Design review of the part built by this model. Coordinates are the model's own, in mm. A direction names the side the tool comes from. Coordinates: 2 decimals unless noted, no trailing zeros. Loops run counter-clockwise (first coordinate to the right, second up) from the corner with the lowest first, then second, coordinate; pieces in that order, holes last. Notation, with made-up numbers: (30, 49.25) - (88, 49.25) arc R19 ccw to (88, 57.25) - close; hole circle Ø10 at (-19.75, 79.25). An arc over 180 degrees is marked (long way). One line per question, with ' | ' between items.
from build123d import *

# Parameters (mm, degrees)
SKETCH_1_W          = 15
SKETCH_1_H          = 15
SKETCH_1_W_2        = 12
SKETCH_1_H_2        = 12
EXTRUDE_1_DEPTH     = 780
CUT_EXTRUDE_1_REACH = 782.288
SKETCH_2_R          = 2.15
CUT_EXTRUDE_2_REACH = 782.288
SKETCH_4_R          = 2.15


with BuildPart() as part:
    # ｽｹｯﾁ1 → 押し出し-薄板1 (new body)
    with BuildSketch(Plane(origin=(0, 0, 0), x_dir=(1, 0, 0), z_dir=(0, 1, 0))):
        with Locations((7.5, 7.5)):
            Rectangle(SKETCH_1_W, SKETCH_1_H)
        with Locations((7.5, 7.5)):
            Rectangle(SKETCH_1_W_2, SKETCH_1_H_2, mode=Mode.SUBTRACT)
    extrude(amount=EXTRUDE_1_DEPTH)

    # ｶｯﾄ - 押し出し1: up to this face of the body (flat: up to its plane)
    cut_extrude_1_end = Plane(part.part.faces().sort_by_distance((0, 390, -7.5))[0])
    # ｽｹｯﾁ2 → ｶｯﾄ - 押し出し1 (cut, up to the picked face)
    with BuildSketch(Plane(origin=(15, 0, 0), x_dir=(0, 0, -1), z_dir=(1, 0, 0)), mode=Mode.PRIVATE) as cut_extrude_1_sk1:
        with Locations((7.5, 730)):
            Circle(SKETCH_2_R)
    cut_extrude_1_tool1 = split(extrude(cut_extrude_1_sk1.sketch, amount=-CUT_EXTRUDE_1_REACH, mode=Mode.PRIVATE), bisect_by=cut_extrude_1_end, keep=Keep.BOTH, mode=Mode.PRIVATE)
    # ｽｹｯﾁ2 → ｶｯﾄ - 押し出し1 (cut, up to the picked face)
    with BuildSketch(Plane(origin=(15, 0, 0), x_dir=(0, 0, -1), z_dir=(1, 0, 0)), mode=Mode.PRIVATE) as cut_extrude_1_sk2:
        with Locations((7.5, 680)):
            Circle(SKETCH_2_R)
    cut_extrude_1_tool2 = split(extrude(cut_extrude_1_sk2.sketch, amount=-CUT_EXTRUDE_1_REACH, mode=Mode.PRIVATE), bisect_by=cut_extrude_1_end, keep=Keep.BOTH, mode=Mode.PRIVATE)
    # ｽｹｯﾁ2 → ｶｯﾄ - 押し出し1 (cut, up to the picked face)
    with BuildSketch(Plane(origin=(15, 0, 0), x_dir=(0, 0, -1), z_dir=(1, 0, 0)), mode=Mode.PRIVATE) as cut_extrude_1_sk3:
        with Locations((7.5, 40)):
            Circle(SKETCH_2_R)
    cut_extrude_1_tool3 = split(extrude(cut_extrude_1_sk3.sketch, amount=-CUT_EXTRUDE_1_REACH, mode=Mode.PRIVATE), bisect_by=cut_extrude_1_end, keep=Keep.BOTH, mode=Mode.PRIVATE)
    # ｽｹｯﾁ2 → ｶｯﾄ - 押し出し1 (cut, up to the picked face)
    with BuildSketch(Plane(origin=(15, 0, 0), x_dir=(0, 0, -1), z_dir=(1, 0, 0)), mode=Mode.PRIVATE) as cut_extrude_1_sk4:
        with Locations((7.5, 770)):
            Circle(SKETCH_2_R)
    cut_extrude_1_tool4 = split(extrude(cut_extrude_1_sk4.sketch, amount=-CUT_EXTRUDE_1_REACH, mode=Mode.PRIVATE), bisect_by=cut_extrude_1_end, keep=Keep.BOTH, mode=Mode.PRIVATE)
    add(cut_extrude_1_tool1.solids().sort_by(Axis((15, 730, -7.5), (-1, 0, 0)))[0], mode=Mode.SUBTRACT)
    add(cut_extrude_1_tool2.solids().sort_by(Axis((15, 680, -7.5), (-1, 0, 0)))[0], mode=Mode.SUBTRACT)
    add(cut_extrude_1_tool3.solids().sort_by(Axis((15, 40, -7.5), (-1, 0, 0)))[0], mode=Mode.SUBTRACT)
    add(cut_extrude_1_tool4.solids().sort_by(Axis((15, 770, -7.5), (-1, 0, 0)))[0], mode=Mode.SUBTRACT)

    # ｶｯﾄ - 押し出し2: up to this face of the body (flat: up to its plane)
    cut_extrude_2_end = Plane(part.part.faces().sort_by_distance((7.5, 390, -15))[0])
    # ｽｹｯﾁ4 → ｶｯﾄ - 押し出し2 (cut, up to the picked face)
    with BuildSketch(Plane.XY, mode=Mode.PRIVATE) as cut_extrude_2_sk1:
        with Locations((7.5, 15)):
            Circle(SKETCH_4_R)
    cut_extrude_2_tool1 = split(extrude(cut_extrude_2_sk1.sketch, amount=-CUT_EXTRUDE_2_REACH, mode=Mode.PRIVATE), bisect_by=cut_extrude_2_end, keep=Keep.BOTH, mode=Mode.PRIVATE)
    # ｽｹｯﾁ4 → ｶｯﾄ - 押し出し2 (cut, up to the picked face)
    with BuildSketch(Plane.XY, mode=Mode.PRIVATE) as cut_extrude_2_sk2:
        with Locations((7.5, 45)):
            Circle(SKETCH_4_R)
    cut_extrude_2_tool2 = split(extrude(cut_extrude_2_sk2.sketch, amount=-CUT_EXTRUDE_2_REACH, mode=Mode.PRIVATE), bisect_by=cut_extrude_2_end, keep=Keep.BOTH, mode=Mode.PRIVATE)
    add(cut_extrude_2_tool1.solids().sort_by(Axis((7.5, 15, 0), (0, 0, -1)))[0], mode=Mode.SUBTRACT)
    add(cut_extrude_2_tool2.solids().sort_by(Axis((7.5, 45, 0), (0, 0, -1)))[0], mode=Mode.SUBTRACT)


solid = part.part
Q1. Draft analysis for pull direction Z (two halves, no side actions). For faces 1 (the flat face through (1.5, 385, -7)), 2 (the flat face through (7, 385, -15)), 3 (the flat face through (15, 385, -7)), state which applies: +Z half, -Z half, draft (parallel to the pull), parting line (faces both ways), or undercut.
Returned:
face 1: undercut | face 2: -Z half | face 3: draft
Q2. For pin 1 (3.5 mm diameter, centred on y = 680, z = -7.5, fed in from +X), flat-tipped, find the tip position at first contact; note if it passes through.
Returned:
pin 1: passes through
Q3. Take a section at A-A (y = 250). Give the boundary of the cut face in (x, z), plus the area to 3 significant figures.
Returned:
outline: (0, -15) - (15, -15) - (15, 0) - (0, 0) - close; hole (1.5, -13.5) - (13.5, -13.5) - (13.5, -1.5) - (1.5, -1.5) - close | area: 81.0 mm²
Q4. Tool access review of faces 4 (the flat face through (7, 385, 0)), 5 (the flat face through (7, 385, -1.5)): name each direction out of +Z, -Z, +X, -X, +Y, -Y from which nothing blocks a thin tool from reaching the whole face with its end or side.
Returned:
face 4: +Z, +X, -X, +Y, -Y | face 5: +Y, -Y
Q5. To check wall thickness, follow line 1 along Y through (x, z) = (14.3, -7.5); line 2 along Y through (x, z) = (7.5, -14.3); line 3 along Z through (x, y) = (1.1, 680). State the ranges of each line that lie inside material, in increasing order.
Returned:
line 1: y = 0 to 37.85, 42.15 to 677.85, 682.15 to 727.85, 732.15 to 767.85, 772.15 to 780 | line 2: y = 0 to 12.85, 17.15 to 42.85, 47.15 to 780 | line 3: z = -15 to -9.65, -5.35 to 0
